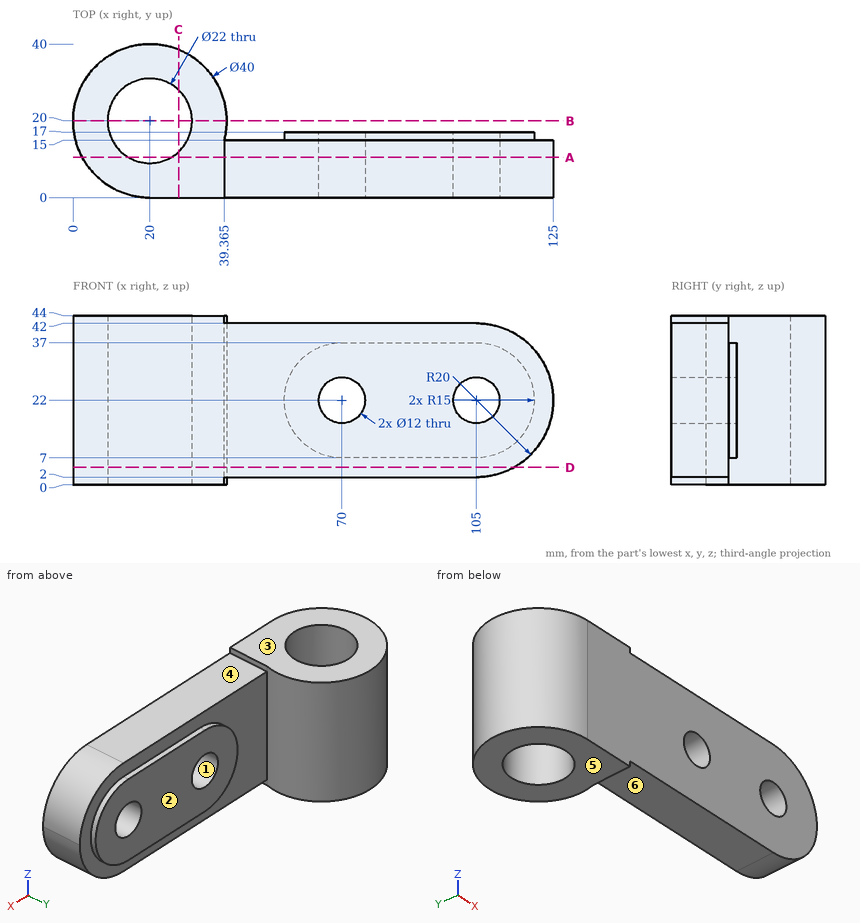
Verification items for this drawing (mm, ordinates from the low corner). A direction names the side the tool comes from. Coordinates: 2 decimals unless noted, no trailing zeros. Loops run counter-clockwise (first coordinate to the right, second up) from the corner with the lowest first, then second, coordinate; pieces in that order, holes last. Notation, with made-up numbers: (-39, 11) -> (16, 11) arc R20 ccw to (16, 42) -> close; hole circle Ø2 at (-23.5, 19). An arc over 180 degrees is marked (long way). Answer in a Markdown table with one row per item. Add a question column.
1. Access from +Z, -Z, +X, -X, +Y, -Y to the whole of each face (thin tool, end or side, straight path). Record for the marked faces 4, 5 and 6.
2. Section check A-A, the plane y = 10.5. Enter the section's corners in (x, z) (3 decimals).
3. Depth check by flat-ended pin: P1, Ø2, axis at x = 89.5, y = 16.5, coming from the +Z side; P2, Ø16.5, axis at x = 76, y = 5, coming from the +Z side; P3, Ø12, axis at y = 5, z = 11, coming from the +X side (3 decimals); P4, Ø17.5, axis at x = 20, y = 20, coming from the -Z side. Enter the tip coordinate at first touch or a pass-through.
4. Draft check along Z on the marked faces 1, 2 and 3. Enter one of: +Z half, -Z half, draft (parallel to the pull), parting line (faces both ways), or undercut.
5. Section check B-B, the plane y = 20. Enter the section's corners in (x, z), then the cut area to 3 significant figures.
6. Section check C-C, the plane x = 27.5. Enter the section's corners in (y, z).
7. Material ranges on probe 1 along Z at (x, y) = (105, 6.5); probe 2 along Y at (x, z) = (20, 31); probe 3 along X at (y, z) = (13.5, 22), recorded low to high. Write a range as [from, to].
8. Section check D-D, the plane z = 4.5. Enter the section's corners in (x, y) (1 decimal), then the cut area to 3 significant figures.
Derived:
| question | item | result |
|---|---|---|
| 1 | face 4 | +Z, +X, +Y, -Y |
| 1 | face 5 | -Z, +X, -X, +Y, -Y |
| 1 | face 6 | -Z, +X, +Y, -Y |
| 2 | outline | (2.4, 0) -> (14.455, 0) -> (14.455, 44) -> (2.4, 44) -> close; (25.545, 0) -> (39.365, 0) -> (39.365, 2) -> (105, 2) arc R20 ccw to (105, 42) -> (39.365, 42) -> (39.365, 44) -> (25.545, 44) -> close; hole circle Ø12 at (70, 22); hole circle Ø12 at (105, 22) |
| 3 | P1 | stops at z = 37 |
| 3 | P2 | stops at z = 42 |
| 3 | P3 | stops at x = 124.365 |
| 3 | P4 | passes through |
| 4 | face 1 | undercut |
| 4 | face 2 | draft |
| 4 | face 3 | +Z half |
| 5 | outline | (0, 0) -> (9, 0) -> (9, 44) -> (0, 44) -> close; (31, 0) -> (40, 0) -> (40, 44) -> (31, 44) -> close |
| 5 | area | 792 mm² |
| 6 | outline | (0, 0) -> (11.95, 0) -> (11.95, 44) -> (0, 44) -> close; (28.05, 0) -> (38.54, 0) -> (38.54, 44) -> (28.05, 44) -> close |
| 7 | probe 1 | z = [2, 16], [28, 42] |
| 7 | probe 2 | y = [0, 9], [31, 40] |
| 7 | probe 3 | x = [1.09, 11.13], [28.87, 64], [76, 99], [111, 125] |
| 8 | outline | (20, 0) -> (114.7, 0) -> (114.7, 15) -> (39.4, 15) arc R20 ccw (long way) to start; hole circle Ø22 at (20, 20) |
| 8 | area | 2,080 mm² |
